Can you work these out from the drawing? Everything is in mm from the part's minimum corner. Round coordinates to 2 decimals unless told otherwise and drop trailing zeros. Write each loop counter-clockwise with the first axis right and the second up, starting at its lowest first coordinate (ties: lowest second). Pieces come first, ordered by that corner, then holes.
Q1. We'd pull the mould along Y, two halves only. Please class the marked faces 1, 2 and 3: +Y half, -Y half, draft (parallel to the pull), parting line (faces both ways), or undercut.
Q2. Please list where these lines run through material, in increasing order: line 1 along Y through (x, z) = (15, 11); line 2 along X through (y, z) = (7.5, 5.25); line 3 along X through (y, z) = (9.5, 2.5).
Q3. If we section it at A-A (x = 12): Please give me the cut outline in (y, z).
Q4. I'm going to push flat-ended pins straight in: pin 1 Ø1.5 at (x, y) = (26, 15) entering from -Z; pin 2 Ø1 at (y, z) = (15.5, 6.5) entering from +X; pin 3 Ø1 at (y, z) = (16.5, 12) entering from +X. Where does each tip first touch, or does it pass through?
Q5. If we section it at B-B (y = 7): Please give me the cut outline in (x, z).
Q6. If we section it at D-D (y = 18.75): Please give me the cut outline in (x, z) (3 decimals), plus the area to 4 significant figures.
Q7. If we section it at C-C (z = 13.5): Please give me the cut outline in (x, y).
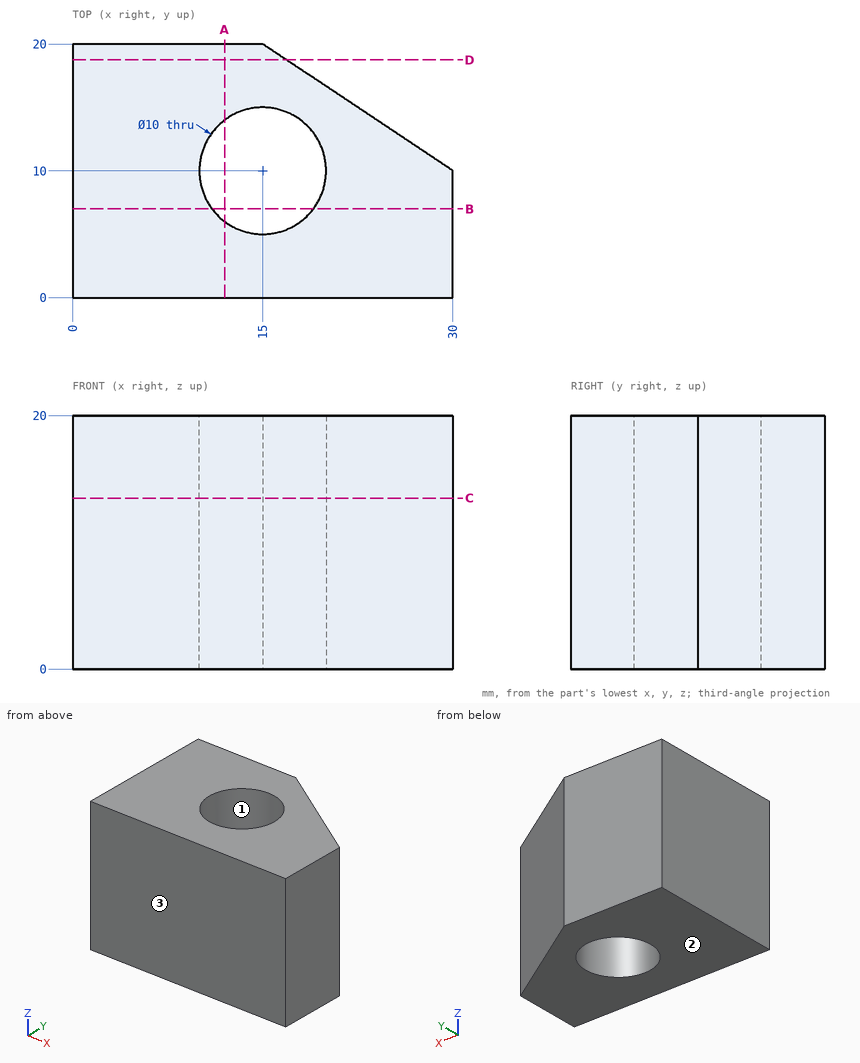
A:
1. face 1: undercut
1. face 2: draft
1. face 3: -Y half
2. line 1: y = 0 to 5, 15 to 20
2. line 2: x = 0 to 10.67, 19.33 to 30
2. line 3: x = 0 to 10.03, 19.97 to 30
3. outline: (0, 0) - (6, 0) - (6, 20) - (0, 20) - close; (14, 0) - (20, 0) - (20, 20) - (14, 20) - close
4. pin 1: passes through
4. pin 2: stops at x = 22.5
4. pin 3: stops at x = 21
5. outline: (0, 0) - (11, 0) - (11, 20) - (0, 20) - close; (19, 0) - (30, 0) - (30, 20) - (19, 20) - close
6. outline: (0, 0) - (16.875, 0) - (16.875, 20) - (0, 20) - close
6. area: 337.5 mm2
7. outline: (0, 0) - (30, 0) - (30, 10) - (15, 20) - (0, 20) - close; hole circle Ø10 at (15, 10)
